from build123d import *

# Parameters (mm, degrees)
SKETCH_1_R      = 4.5
SKETCH_1_R_2    = 1.25
SKETCH_1_W      = 12.5
SKETCH_1_H      = 22.8
EXTRUDE_1_DEPTH = 3
EXTRUDE_START   = 20
SKETCH_3_R      = 1.1
SKETCH_3_R_2    = 1.5
EXTRUDE_2_DEPTH = 3
SKETCH_4_R      = 7.5
SKETCH_4_R_2    = 4.5
EXTRUDE_3_DEPTH = 7
EXTRUDE_START_2 = 7
SKETCH_5_R      = 10
SKETCH_5_R_2    = 7.5
EXTRUDE_4_DEPTH = 7


with BuildPart() as part:
    # 草图1 → 凸台-拉伸1 (new body)
    with BuildSketch(Plane(origin=(0, 0, 0), x_dir=(1, 0, 0), z_dir=(0, 1, 0))):
        with BuildLine():
            Line((-20, -15.9), (20, -15.9))
            Line((20, -15.9), (20, 10.9))
            ThreePointArc((20, 10.9), (17.949747468, 15.849747468), (13, 17.9))
            Line((13, 17.9), (-13, 17.9))
            ThreePointArc((-13, 17.9), (-17.949747468, 15.849747468), (-20, 10.9))
            Line((-20, 10.9), (-20, -15.9))
        make_face()
        with Locations(Location((-10, 5.2, 0), (0, 0, 270))):
            Circle(SKETCH_1_R, mode=Mode.SUBTRACT)
        with Locations(Location((10, 13.85, 0), (0, 0, 270))):
            Circle(SKETCH_1_R_2, mode=Mode.SUBTRACT)
        with Locations(Location((10, -13.85, 0), (0, 0, 270))):
            Circle(SKETCH_1_R_2, mode=Mode.SUBTRACT)
        with Locations((10, 0)):
            Rectangle(SKETCH_1_W, SKETCH_1_H, mode=Mode.SUBTRACT)
    extrude(amount=EXTRUDE_1_DEPTH)

    # 草图3 → 凸台-拉伸2 (add)
    with BuildSketch(Plane(origin=(0, 0, 0), x_dir=(0, 0, -1), z_dir=(1, 0, 0)).offset(EXTRUDE_START)):
        with BuildLine():
            Line((-15.9, 3), (-15.9, 23))
            Line((-15.9, 23), (-34.9, 23))
            ThreePointArc((-34.9, 23), (-44.9, 33), (-34.9, 43))
            Line((-34.9, 43), (-5.9, 43))
            Line((-5.9, 43), (-5.9, 13))
            Line((-5.9, 13), (10.9, 13))
            Line((10.9, 13), (10.9, 3))
            Line((10.9, 3), (-15.9, 3))
        make_face()
        with Locations(Location((-42.15, 33, 0), (0, 0, 180))):
            Circle(SKETCH_3_R, mode=Mode.SUBTRACT)
        with Locations(Location((-34.9, 40.25, 0), (0, 0, 180))):
            Circle(SKETCH_3_R, mode=Mode.SUBTRACT)
        with Locations(Location((-27.65, 33, 0), (0, 0, 180))):
            Circle(SKETCH_3_R, mode=Mode.SUBTRACT)
        with Locations(Location((-34.9, 25.75, 0), (0, 0, 180))):
            Circle(SKETCH_3_R, mode=Mode.SUBTRACT)
        with Locations(Location((-34.9, 33, 0), (0, 0, 180))):
            Circle(SKETCH_3_R_2, mode=Mode.SUBTRACT)
    extrude(amount=-EXTRUDE_2_DEPTH)

    # 草图4 → 凸台-拉伸3 (add)
    with BuildSketch(Plane(origin=(0, 3, 0), x_dir=(1, 0, 0), z_dir=(0, 1, 0))):
        with Locations(Location((-10, 5.2, 0), (0, 0, 90))):
            Circle(SKETCH_4_R)
        with Locations(Location((-10, 5.2, 0), (0, 0, 270))):
            Circle(SKETCH_4_R_2, mode=Mode.SUBTRACT)
    extrude(amount=EXTRUDE_3_DEPTH)

    # 草图5 → 凸台-拉伸4 (add)
    with BuildSketch(Plane.XZ.offset(EXTRUDE_START_2)):
        with Locations(Location((-10, -5.2, 0), (0, 0, 180))):
            Circle(SKETCH_5_R)
        with Locations(Location((-10, -5.2, 0), (0, 0, 270))):
            Circle(SKETCH_5_R_2, mode=Mode.SUBTRACT)
    extrude(amount=-EXTRUDE_4_DEPTH)


solid = part.part
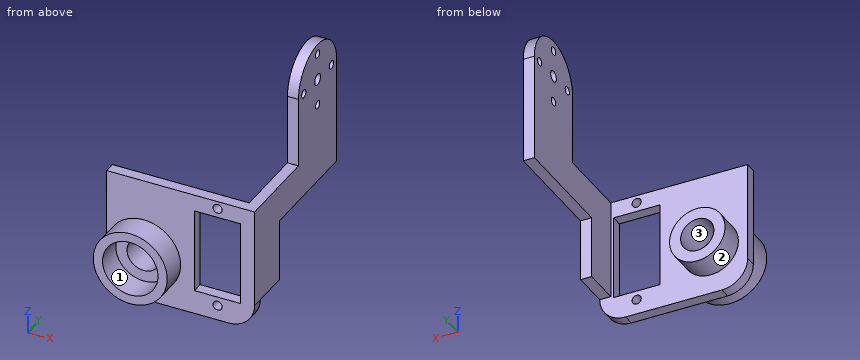
Source: CAD feature listing. Evaluate the final solid. Frame: model axes, mm. Face numbers are marked on the shaded views. A direction names the side the tool comes from. Coordinates: 2 decimals unless noted, no trailing zeros. Loops run counter-clockwise (first coordinate to the right, second up) from the corner with the lowest first, then second, coordinate; pieces in that order, holes last. Notation, with made-up numbers: (63, -13.75) -> (67, -13.75) arc R28 ccw to (67, 9.25) -> close; hole circle Ø7 at (-7.5, 23.5). An arc over 180 degrees is marked (long way). Answer in a Markdown table with one row per item. Add a question column.
Q1. Contact query for flat-ended pins moving along their axis: pin 1 Ø3.5 at (y, z) = (33, 34.9) entering from -X; pin 2 Ø13.5 at (x, z) = (-10, -5.2) entering from -Y; pin 3 Ø6 at (x, z) = (-0.5, -8) entering from +Y. Output: stop coordinate, or through.
Q2. Section D-D on y = 9. Return the cut outline in (x, z), and give its area (3 significant figures).
Q3. Section B-B on x = 10. Return the cut outline in (y, z), and give its area (3 significant figures).
Q4. Section A-A on y = 33. Return the cut outline in (x, z), and give its area (3 significant figures).
Q5. Reachability of the marked faces 1, 2 and 3 from +Z, -Z, +X, -X, +Y, -Y: full face, straight path, thin tool, end or side. Return the list, or none.
Q6. Section C-C on z = 27.65. Return the cut outline in (x, y), and give its area (3 significant figures).
Q7. Ray query, line 1 along Z through (x, y) = (18.25, 33); line 2 along Y through (x, z) = (18.75, 34.9); line 3 along Y through (x, z) = (17, -13). Return the intervals inside material, ascending.
Computed values:
| question | item | result |
|---|---|---|
| 1 | pin 1 | stops at x = 17 |
| 1 | pin 2 | stops at y = 0 |
| 1 | pin 3 | stops at y = 10 |
| 2 | outline | circle Ø15 at (-10, -5.2); (17, -10.9) -> (20, -10.9) -> (20, 15.9) -> (17, 15.9) -> close; hole circle Ø9 at (-10, -5.2) |
| 2 | area | 193 mm^2 |
| 3 | outline | (0, -17.9) -> (3, -17.9) -> (3, -15.1) -> (0, -15.1) -> close; (0, -12.6) -> (3, -12.6) -> (3, -11.4) -> (0, -11.4) -> close; (0, 11.4) -> (3, 11.4) -> (3, 12.6) -> (0, 12.6) -> close; (0, 15.1) -> (3, 15.1) -> (3, 15.9) -> (0, 15.9) -> close |
| 3 | area | 18.0 mm^2 |
| 4 | outline | (17, 5.9) -> (20, 5.9) -> (20, 26.55) -> (17, 26.55) -> close; (17, 28.75) -> (20, 28.75) -> (20, 33.4) -> (17, 33.4) -> close; (17, 36.4) -> (20, 36.4) -> (20, 41.05) -> (17, 41.05) -> close; (17, 43.25) -> (20, 43.25) -> (20, 44.9) -> (17, 44.9) -> close |
| 4 | area | 94.8 mm^2 |
| 5 | face 1 | -Y |
| 5 | face 2 | +Y |
| 5 | face 3 | +Y, -Y |
| 6 | outline | (17, 23) -> (20, 23) -> (20, 31.9) -> (17, 31.9) -> close; (17, 34.1) -> (20, 34.1) -> (20, 43) -> (17, 43) -> close |
| 6 | area | 53.4 mm^2 |
| 7 | line 1 | z = 5.9 to 26.55, 28.75 to 33.4, 36.4 to 41.05, 43.25 to 44.9 |
| 7 | line 2 | y = 23 to 24.65, 26.85 to 31.5, 34.5 to 39.15, 41.35 to 43 |
| 7 | line 3 | y = 0 to 3 |
